Design review of the part built by this model. Coordinates are the model's own, in mm. A direction names the side the tool comes from. Give positions to 0.01 mm unless a question says otherwise; leave off trailing zeros. Loops run counter-clockwise (first coordinate to the right, second up) from the corner with the lowest first, then second, coordinate; pieces in that order, holes last. Notation, with made-up numbers: (37.5, 61) -> (53.5, 61) arc R35 cw to (53.5, 98) -> close; hole circle Ø3 at (-20, 21.5). An arc over 180 degrees is marked (long way). Use CSV: the item, a comma, the result in double quotes. Start each with the question number.
Item 1: For faces 4 (the face through (5.42, -4.894, 4.436)), 5 (the face through (-38.217, 0, 2)), 6 (the face through (-2.21, 3.18, 4.44)), 7 (the face through (15.055, -5.436, 4.436)), list the 3-axis set-ups (+Z, -Z, +X, -X, +Y, -Y) from which the entire face can be reached by the end or side of a thin tool; tool diameter is ignored.
Item 2: Wall thickness on line 1 along Y through (x, z) = (32.5, 4.25); line 2 along X through (y, z) = (1.5, 0.7); line 3 along Z through (x, y) = (32.5, -11): over which ranges is each line inside the solid? List them lowest first. Write a range as from..to.
Item 3: We need section C-C (x = -9.5). State the section outline as (y, z) points.
Item 4: The part is to be moulded in two halves that separate along Y. For faces 1 (the face through (43.545, 10.951, 1.878)), 2 (the face through (-7, 0.3, 3.81)), 3 (the face through (43.495, -11.001, 1.878)), say which applies: +Y half, -Y half, draft (parallel to the pull), parting line (faces both ways), or undercut.
Item 5: We need section B-B (x = 19.5). State the section outline as (y, z) points, plus the area to 3 significant figures.
Item 6: We need section A-A (z = 2.45). State the section outline as (x, y) points (3 decimals), plus the area to 3 significant figures.
Item 7: Clearance check with flat-ended pins moving along their axes: pin 1 (1 mm diameter, centred on y = 3.5, z = 4.5, fed in from +X); pin 2 (1 mm diameter, centred on x = 32, z = 4.5, fed in from -Y); pin 3 (2 mm diameter, centred on x = 26.5, z = 4, fed in from -Y); pin 4 (0.6 mm diameter, centred on y = -0.5, z = 4.5, fed in from +X). State where each tip first meets the part, or that it passes through.
from build123d import *

# Parameters (mm, degrees)
F1_DEPTH = 3.81
F3_DEPTH = 1.27


with BuildPart() as f1:
    # F0 (on Top) → F1 (new body)
    with BuildSketch(Plane.XY):
        with BuildLine():
            Line((-41.275, -11.90625), (41.275, -11.90625))
            ThreePointArc((41.275, -11.90625), (43.5200640303, -10.9763140303), (44.45, -8.73125))
            Line((44.45, -8.73125), (44.45, 8.73125))
            ThreePointArc((44.45, 8.73125), (43.5200640303, 10.9763140303), (41.275, 11.90625))
            Line((41.275, 11.90625), (-41.275, 11.90625))
            ThreePointArc((-41.275, 11.90625), (-43.5200640303, 10.9763140303), (-44.45, 8.73125))
            Line((-44.45, 8.73125), (-44.45, -8.73125))
            ThreePointArc((-44.45, -8.73125), (-43.5200640303, -10.9763140303), (-41.275, -11.90625))
        make_face()
        with BuildLine():
            Line((-38.2169688356, 4.445), (-38.2169688356, -4.445))
            ThreePointArc((-38.2169688356, -4.445), (-38.7749304174, -5.7920384182), (-40.1219688356, -6.35))
            ThreePointArc((-40.1219688356, -6.35), (-41.4690072538, -5.7920384182), (-42.0269688356, -4.445))
            Line((-42.0269688356, -4.445), (-42.0269688356, 4.445))
            ThreePointArc((-42.0269688356, 4.445), (-41.4690072538, 5.7920384182), (-40.1219688356, 6.35))
            ThreePointArc((-40.1219688356, 6.35), (-38.7749304174, 5.7920384182), (-38.2169688356, 4.445))
        make_face(mode=Mode.SUBTRACT)
    extrude(amount=F1_DEPTH)

    # F2 (on face) → F3 (join)
    with BuildSketch(Plane.XY.offset(3.81)):
        with BuildLine():
            Line((-33.1369688356, 8.09625), (-33.1369688356, -8.09625))
            Line((-33.1369688356, -8.09625), (-14.9305017963, -8.09625))
            Line((-14.9305017963, -8.09625), (-4.4408244503, -8.09625))
            Line((-4.4408244503, -8.09625), (-4.4408244503, -6.06425))
            Line((-4.4408244503, -6.06425), (-14.7659257054, -6.06425))
            add(Edge.make_bspline(
                [(-13.513635844, -2.032), (-13.8611532829, -2.1980739704), (-14.3459285269, -2.2099492601), (-14.4823312004, -4.002820532), (-14.7172564306, -5.3877740164), (-14.7775029403, -5.761799907), (-14.7659257054, -6.06425)],
                knots=[0, 0, 0, 0, 0.2107594837, 0.5139383753, 0.8003027815, 1, 1, 1, 1], degree=3))
            Line((-13.513635844, -2.032), (-6.8832325343, -2.032))
            Line((-6.8832325343, -2.032), (-6.8832325343, 0))
            Line((-6.8832325343, 0), (-13.9832440764, 0))
            add(Edge.make_bspline(
                [(-11.374309659, 6.06425), (-11.7970469078, 6.0937481421), (-12.400656261, 6.0408242331), (-12.9628712261, 4.3407982551), (-13.3836406147, 2.9409234174), (-13.8567248974, 1.0073529425), (-13.9832440764, 0)],
                knots=[0, 0, 0, 0, 0.1854469036, 0.4247933811, 0.6668574102, 1, 1, 1, 1], degree=3))
            Line((-11.374309659, 6.06425), (-5.4148057359, 6.06425))
            Line((-5.4148057359, 6.06425), (-5.4148057359, 6.5723256238))
            Line((-5.4148057359, 6.5723256238), (-5.4148057359, 8.09625))
            Line((-5.4148057359, 8.09625), (-13.4092783555, 8.09625))
            add(Edge.make_bspline(
                [(-17.6879316568, -0.762), (-17.0853493776, 1.2922751779), (-16.7349072936, 2.3189827137), (-15.8911126674, 4.4121063422), (-15.0710282171, 6.5370694937), (-14.3847178975, 7.6672909404), (-13.9179741964, 8.0772032961), (-13.4092783555, 8.09625)],
                knots=[0, 0, 0, 0, 0.2707299894, 0.4717983457, 0.6911291675, 0.8524377102, 1, 1, 1, 1], degree=3))
            Line((-17.6879316568, -0.762), (-15.3005402535, -0.762))
            add(Edge.make_bspline(
                [(-17.6879316568, -6.06425), (-17.5631227568, -5.0804670724), (-17.5265823635, -5.0281161064), (-17.1728408985, -3.2023736826), (-16.8475061728, -2.1905918672), (-16.1243397189, -1.1537855527), (-15.7725399015, -0.9954859224), (-15.3005402535, -0.762)],
                knots=[0, 0, 0, 0, 0.2097857454, 0.4327627354, 0.6303900109, 0.8195013475, 1, 1, 1, 1], degree=3))
            Line((-17.6879316568, -6.06425), (-30.5969688356, -6.06425))
            Line((-30.5969688356, -6.06425), (-30.5969688356, 8.09625))
            Line((-30.5969688356, 8.09625), (-33.1369688356, 8.09625))
        make_face()
        Polygon((-4.4408244503, -6.06425), (-4.4408244503, -8.09625), (-3.57352963, -8.09625), (2.4774279686, -1.7803364764), (1.0801424445, -0.3015341148), align=None)
        Polygon((2.8394880429, 1.5348487183), (1.0801424445, -0.3015341148), (2.4774279686, -1.7803364764), (4.2367735671, 0.0560463568), align=None)
        Polygon((-5.4148057359, 6.5723256238), (1.0801424445, -0.3015341148), (2.8394880429, 1.5348487183), (-3.3602255002, 8.09625), (-5.4148057359, 8.09625), align=None)
        Polygon((4.2367735671, 0.0560463568), (2.4774279686, -1.7803364764), (8.4451859107, -8.09625), (11.9396863995, -8.09625), align=None)
        Polygon((9.1256350578, 8.09625), (2.8394880429, 1.5348487183), (4.2367735671, 0.0560463568), (11.3477446789, 7.4783886686), (11.9396863995, 8.09625), align=None)
        with BuildLine():
            Line((11.9396863995, 8.09625), (11.3477446789, 7.4783886686))
            Line((11.3477446789, 7.4783886686), (11.3477446789, -4.3666326941))
            ThreePointArc((11.3477446789, -4.3666326941), (12.4013025669, -6.9070776733), (14.9435433322, -7.9562949086))
            Line((14.9435433322, -7.9562949086), (24.6688841279, -7.9396838649))
            Line((24.6688841279, -7.9396838649), (24.6688841279, -5.9076838649))
            Line((24.6688841279, -5.9076838649), (24.6688841279, 8.09625))
            Line((24.6688841279, 8.09625), (22.6368841279, 8.09625))
            Line((22.6368841279, 8.09625), (22.6368841279, -6.3459635714))
            Line((22.6368841279, -6.3459635714), (17.4303608148, -6.3459635714))
            ThreePointArc((17.4303608148, -6.3459635714), (15.0273352941, -5.4111473397), (13.8877446789, -3.0981954877))
            Line((13.8877446789, -3.0981954877), (13.8877446789, 8.09625))
            Line((13.8877446789, 8.09625), (11.9396863995, 8.09625))
        make_face()
        with BuildLine():
            Line((24.6688841279, -5.9076838649), (24.6688841279, -7.9396838649))
            Line((24.6688841279, -7.9396838649), (37.8373786807, -7.9396838649))
            add(Edge.make_bspline(
                [(37.8373786807, -7.9396838649), (38.4882097852, -7.8114506673), (39.5178452641, -7.496112843), (40.126883642, -6.0991216047), (40.7050802618, -4.8496198201), (40.5764483682, -3.0792560488), (39.7269584552, -1.6891831447), (38.8078867235, -0.737734011), (37.8093798081, -0.2945075978), (36.4599787891, 0.0450284712), (34.7408936011, 0.1986066109), (34.1846869754, 0.1883161351)],
                knots=[0, 0, 0, 0, 0.1171066483, 0.2235125119, 0.3294259119, 0.4469201861, 0.5621007917, 0.6644797625, 0.7558675462, 0.8648976622, 1, 1, 1, 1], degree=3))
            Line((34.1846869754, 0.1883161351), (29.2448235171, 0.1883161351))
            add(Edge.make_bspline(
                [(29.2448235171, 0.1883161351), (29.4537920477, 0.9562330478), (29.3473473778, 2.6260589886), (30.233558549, 4.9044254628), (31.1930093172, 5.7724721465), (32.0247337222, 6.06425)],
                knots=[0, 0, 0, 0, 0.3448282666, 0.6791586925, 1, 1, 1, 1], degree=3))
            Line((32.0247337222, 6.06425), (41.9643558562, 6.06425))
            Line((41.9643558562, 6.06425), (41.9643558562, 8.09625))
            Line((41.9643558562, 8.09625), (33.1864038537, 8.09625))
            add(Edge.make_bspline(
                [(25.4828148948, -1.8436838649), (25.680435092, -1.0761085159), (26.0689778517, -0.0750567317), (26.6999114572, 2.5205566329), (27.6657264028, 4.9797411998), (29.0563776932, 7.0524197018), (30.311457036, 7.7653827779), (31.6423733416, 8.1991717396), (32.7591321523, 8.0866993991), (33.1864038537, 8.09625)],
                knots=[0, 0, 0, 0, 0.1419463815, 0.3049859755, 0.4748327911, 0.63374866, 0.7540605138, 0.8743708506, 1, 1, 1, 1], degree=3))
            Line((25.4828148948, -1.8436838649), (35.8053786807, -1.8436838649))
            ThreePointArc((35.8053786807, -1.8436838649), (37.2422196601, -2.4388428856), (37.8373786807, -3.8756838649))
            ThreePointArc((37.8373786807, -3.8756838649), (37.2422196601, -5.3125248443), (35.8053786807, -5.9076838649))
            Line((35.8053786807, -5.9076838649), (24.6688841279, -5.9076838649))
        make_face()
    extrude(amount=F3_DEPTH)


solid = f1.part
Results found:
1,face 4,"+Z, -Y"
1,face 5,"+Z, -Z"
1,face 6,"+Z"
1,face 7,"+Z, +Y"
2,line 1,"-7.94..-5.91, -1.84..0.19, 6.06..8.11"
2,line 2,"-44.45..-42.03, -38.22..44.45"
2,line 3,"0..3.81"
3,outline,"(-11.91, 0) -> (11.91, 0) -> (11.91, 3.81) -> (8.1, 3.81) -> (8.1, 5.08) -> (6.06, 5.08) -> (6.06, 3.81) -> (0, 3.81) -> (0, 5.08) -> (-2.03, 5.08) -> (-2.03, 3.81) -> (-6.06, 3.81) -> (-6.06, 5.08) -> (-8.1, 5.08) -> (-8.1, 3.81) -> (-11.91, 3.81) -> close"
4,face 1,"+Y half"
4,face 2,"undercut"
4,face 3,"-Y half"
5,outline,"(-11.91, 0) -> (11.91, 0) -> (11.91, 3.81) -> (-6.35, 3.81) -> (-6.35, 5.08) -> (-7.95, 5.08) -> (-7.95, 3.81) -> (-11.91, 3.81) -> close"
5,area,"92.8 mm²"
6,outline,"(-44.45, -8.731) arc R3.175 ccw to (-41.275, -11.906) -> (41.275, -11.906) arc R3.175 ccw to (44.45, -8.731) -> (44.45, 8.731) arc R3.175 ccw to (41.275, 11.906) -> (-41.275, 11.906) arc R3.175 ccw to (-44.45, 8.731) -> close; hole (-42.027, -4.445) arc R1.905 ccw to (-38.217, -4.445) -> (-38.217, 4.445) arc R1.905 ccw to (-42.027, 4.445) -> close"
6,area,"2,060 mm²"
7,pin 1,"x = 29.93"
7,pin 2,"y = -7.94"
7,pin 3,"y = -11.91"
7,pin 4,"x = 38.77"
